Verification items for the finished model (mm, model axes). Face numbers are marked on the shaded views. A direction names the side the tool comes from. Coordinates: 2 decimals unless noted, no trailing zeros. Write each loop counter-clockwise with the first axis right and the second up, starting at its lowest first coordinate (ties: lowest second). Pieces come first, ordered by that corner, then holes. Notation, with made-up numbers: (-0.75, 71) -> (57.25, 71) arc R14 cw to (57.25, 93) -> close; hole circle Ø2 at (67.25, 70.25). An arc over 180 degrees is marked (long way). Answer in a Markdown table with one row per item.
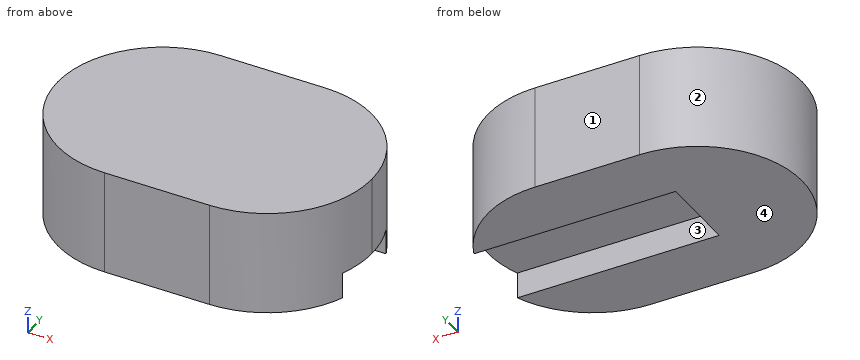
```python
from build123d import *

# Parameters (mm, degrees)
F1_DEPTH = 12.7
F3_DEPTH = 3.175


with BuildPart() as f1:
    # F0 (on Top) → F1 (new body)
    with BuildSketch(Plane.XY):
        with BuildLine():
            Line((0, 0), (0, 12.7))
            ThreePointArc((0, 12.7), (-12.7, 0), (0, -12.7))
            Line((0, -12.7), (0, 0))
        make_face()
        with BuildLine():
            Line((12.7, 0), (0, 0))
            ThreePointArc((0, 0), (1.701477, -6.35), (6.35, -10.998523))
            ThreePointArc((6.35, -10.998523), (10.998523, -6.35), (12.7, 0))
        make_face()
        with BuildLine():
            Line((0, 0), (0, -12.7))
            ThreePointArc((0, -12.7), (3.287002, -12.267258), (6.35, -10.998523))
            ThreePointArc((6.35, -10.998523), (1.701477, -6.35), (0, 0))
        make_face()
        with BuildLine():
            ThreePointArc((6.35, 10.998523), (3.287002, 12.267258), (0, 12.7))
            Line((0, 12.7), (0, 0))
            ThreePointArc((0, 0), (1.701477, 6.35), (6.35, 10.998523))
        make_face()
        with BuildLine():
            ThreePointArc((12.7, 0), (10.998523, 6.35), (6.35, 10.998523))
            ThreePointArc((6.35, 10.998523), (1.701477, 6.35), (0, 0))
            Line((0, 0), (12.7, 0))
        make_face()
        with BuildLine():
            ThreePointArc((12.7, 12.7), (9.412998, 12.267258), (6.35, 10.998523))
            ThreePointArc((6.35, 10.998523), (10.998523, 6.35), (12.7, 0))
            Line((12.7, 0), (12.7, 12.7))
        make_face()
        with BuildLine():
            ThreePointArc((25.4, 0), (21.680256, 8.980256), (12.7, 12.7))
            Line((12.7, 12.7), (12.7, 0))
            Line((12.7, 0), (12.7, -12.7))
            ThreePointArc((12.7, -12.7), (21.680256, -8.980256), (25.4, 0))
        make_face()
        with BuildLine():
            ThreePointArc((6.35, -10.998523), (3.287002, -12.267258), (0, -12.7))
            Line((0, -12.7), (12.7, -12.7))
            ThreePointArc((12.7, -12.7), (9.412998, -12.267258), (6.35, -10.998523))
        make_face()
        with BuildLine():
            Line((12.7, 12.7), (0, 12.7))
            ThreePointArc((0, 12.7), (3.287002, 12.267258), (6.35, 10.998523))
            ThreePointArc((6.35, 10.998523), (9.412998, 12.267258), (12.7, 12.7))
        make_face()
        with BuildLine():
            ThreePointArc((12.7, 0), (10.998523, -6.35), (6.35, -10.998523))
            ThreePointArc((6.35, -10.998523), (9.412998, -12.267258), (12.7, -12.7))
            Line((12.7, -12.7), (12.7, 0))
        make_face()
    extrude(amount=F1_DEPTH)

    # F2 (on Top) → F3 (cut)
    with BuildSketch(Plane.XY):
        Polygon((0, 4.7625), (0, 0), (0, -4.7625), (25.4, -4.7625), (25.4, 4.7625), align=None)
    extrude(amount=F3_DEPTH, mode=Mode.SUBTRACT)


solid = f1.part
```
1. Section check C-C, the plane y = -2.5. Record the boundary of the cut face in (x, z) (1 decimal), plus the area to 3 significant figures.
Geometry says:
| item | result |
|---|---|
| outline | (-12.5, 0) -> (0, 0) -> (0, 3.2) -> (25.2, 3.2) -> (25.2, 12.7) -> (-12.5, 12.7) -> close |
| area | 398 mm^2 |
2. Tool access check on the marked faces 3 and 4. Record the directions out of +Z, -Z, +X, -X, +Y, -Y that give a thin tool (end or side, any length) a straight path to the whole face; none if there is none.
Geometry says:
| item | result |
|---|---|
| face 3 | -Z, +X |
| face 4 | -Z, +X, -X, +Y, -Y |
3. Section check B-B, the plane z = 2.75. Record the boundary of the cut face in (x, y), plus the area to 3 significant figures.
Geometry says:
| item | result |
|---|---|
| outline | (0, -12.7) -> (12.7, -12.7) arc R12.7 ccw to (24.47, -4.76) -> (0, -4.76) -> (0, 4.76) -> (24.47, 4.76) arc R12.7 ccw to (12.7, 12.7) -> (0, 12.7) arc R12.7 ccw to start |
| area | 590 mm^2 |
4. Thickness scan on line 1 (Y direction, x = 13, z = 6); line 2 (Z direction, x = 11, y = 3.75) (3 decimals); line 3 (X direction, y = -0.25, z = 8.25). Record the ranges inside material, lowest first. Write a range as from..to.
Geometry says:
| item | result |
|---|---|
| line 1 | -12.7..12.7 |
| line 2 | 3.175..12.7 |
| line 3 | -12.7..25.4 |
5. Section check A-A, the plane x = 9. Record the boundary of the cut face in (y, z) (1 decimal), plus the area to 3 significant figures.
Geometry says:
| item | result |
|---|---|
| outline | (-12.7, 0) -> (-4.8, 0) -> (-4.8, 3.2) -> (4.8, 3.2) -> (4.8, 0) -> (12.7, 0) -> (12.7, 12.7) -> (-12.7, 12.7) -> close |
| area | 292 mm^2 |
6. Depth check by flat-ended pin: P1, Ø1, axis at x = 18, z = 1, coming from the -Y side; P2, Ø1, axis at y = 3.5, z = 5, coming from the +X side; P3, Ø1, axis at x = 15.5, z = 1, coming from the +Y side; P4, Ø12, axis at x = -6.5, y = -4.5, coming from the -Z side. Enter the tip coordinate at first touch or a pass-through.
Geometry says:
| item | result |
|---|---|
| P1 | y = -11.76 |
| P2 | x = 25.04 |
| P3 | y = 12.49 |
| P4 | z = 0 |
7. Section check D-D, the plane x = -2.5. Record the boundary of the cut face in (y, z).
Geometry says:
| item | result |
|---|---|
| outline | (-12.45, 0) -> (12.45, 0) -> (12.45, 12.7) -> (-12.45, 12.7) -> close |
8. Mould release check, pull along X, two halves, no side actions. Record for the marked faces 1 and 2: released by +X, released by -X, zero draft, split by the parting line, or undercut.
Geometry says:
| item | result |
|---|---|
| face 1 | zero draft |
| face 2 | released by -X |
